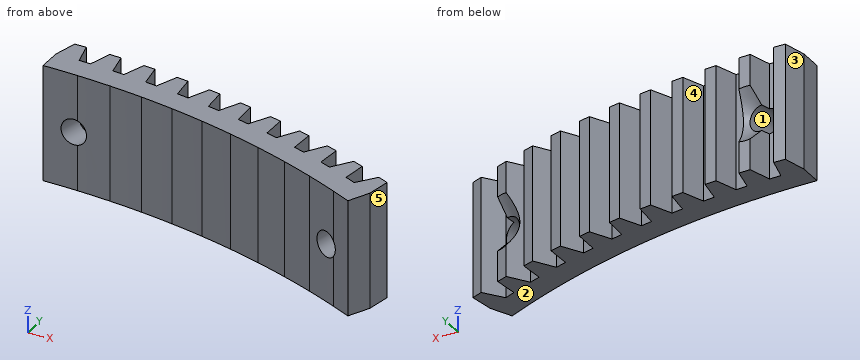
from build123d import *

# Parameters (mm, degrees)
BOSS_EXTRUDE1_DEPTH                                = 25.4
CIRPATTERN2_COUNT                                  = 11
CIRPATTERN2_ANGLE                                  = 23.5
CUT_EXTRUDE2_DEPTH                                 = 25.4
CSK_FOR_10_FLAT_HEAD_MACHINE_SCREW_100_D           = 5.6134
CSK_FOR_10_FLAT_HEAD_MACHINE_SCREW_100_CSINK_D     = 12.7
CSK_FOR_10_FLAT_HEAD_MACHINE_SCREW_100_CSINK_ANGLE = 90


with BuildPart() as part:
    # Sketch1 → Boss-Extrude1 (new body)
    with BuildSketch(Plane.XY):
        with BuildLine():
            Line((1.27, 190.5), (0, 185.42))
            Line((0, 185.42), (0, 180.34))
            ThreePointArc((0, 180.34), (3.828563565, 180.299355798), (7.655401402, 180.177441511))
            Line((7.655401402, 180.177441511), (7.874, 185.32237567))
            ThreePointArc((7.874, 185.32237567), (6.477183927, 185.376451817), (5.08, 185.42))
            Line((5.08, 185.42), (3.81, 190.5))
            Line((3.81, 190.5), (1.27, 190.5))
        make_face()
    boss_extrude1 = extrude(amount=BOSS_EXTRUDE1_DEPTH)

    # CirPattern2: Boss-Extrude1 ×11 about axis
    cirpattern2_axis = Axis((0, 0, 0), (0, 0, -1))
    for i in range(1, CIRPATTERN2_COUNT):
        add(boss_extrude1.rotate(cirpattern2_axis, i * CIRPATTERN2_ANGLE / (CIRPATTERN2_COUNT - 1)))

    # Sketch4 → Cut-Extrude2 (cut)
    with BuildSketch(Plane.XY.offset(25.4)):
        with BuildLine():
            Line((78.866050023, 162.180953733), (81.118055775, 166.812001449))
            ThreePointArc((81.118055775, 166.812001449), (79.858654337, 167.418571633), (78.594717538, 168.015633722))
            Line((78.594717538, 168.015633722), (76.34244866, 163.384044914))
            ThreePointArc((76.34244866, 163.384044914), (77.606580732, 162.787389644), (78.866050023, 162.180953733))
        make_face()
    extrude(amount=-CUT_EXTRUDE2_DEPTH, mode=Mode.SUBTRACT)

    # CSK for _10 Flat Head Machine Screw _100 (through all)
    with Locations(Plane(origin=(40.80368391, 183.714401712, 0), x_dir=(-0.976211516, 0.216820379, 0), z_dir=(0.216820379, 0.976211516, 0))):
        with Locations((-32.344274852, 12.7), (32.394112766, 12.7)):
            CounterSinkHole(CSK_FOR_10_FLAT_HEAD_MACHINE_SCREW_100_D / 2, CSK_FOR_10_FLAT_HEAD_MACHINE_SCREW_100_CSINK_D / 2, counter_sink_angle=CSK_FOR_10_FLAT_HEAD_MACHINE_SCREW_100_CSINK_ANGLE)


solid = part.part
Input: part model. Units: mm. Frame: model coordinates. Face numbers are marked on the shaded views. A direction names the side the tool comes from. Coordinates: 2 decimals unless noted, no trailing zeros. Order: outer loops, then holes, each group sorted by start corner. A loop starts at its lowest first (then second) coordinate and runs counter-clockwise, first axis right, second up.
1. Access query for the marked faces 4 and 5. Directions: +Z, -Z, +X, -X, +Y, -Y. A direction counts if a zero-diameter tool reaches every point of the face in a straight line with its end or side. Return the directions, or none.
Checked values:
face 4: +Z, -Z, +Y
face 5: +Z, -Z, +X, -Y
2. Cut plane B-B, the plane x = 34. Return loops of the section in (y, z), plus the area to 3 significant figures.
Checked values:
outline: (177.11, 0) - (187.46, 0) - (187.46, 25.4) - (177.11, 25.4) - close
area: 263 mm2
3. Contact query for flat-ended pins moving along their axis: P1, Ø4, axis at x = 54, y = 184.5, coming from the +Z side (1 decimal); P2, Ø3, axis at y = 167, z = 7.5, coming from the +X side; P3, Ø8, axis at x = 47.5, z = 5.5, coming from the +Y side; P4, Ø3, axis at y = 180.5, z = 9.5, coming from the -X side. Output: stop coordinate, or through.
Checked values:
P1: passes through
P2: stops at x = 78.68
P3: stops at y = 184.45
P4: stops at x = 0
4. Draft query along Z for the marked faces 1, 2 and 3. Return one class per face: +Z half, -Z half, draft (parallel to the pull), parting line (faces both ways), or undercut.
Checked values:
face 1: undercut
face 2: -Z half
face 3: draft
5. Cut plane A-A, the plane z = 13.5. Count the separate pieces of the cut face and the enclosed holes in it, plus the area to 3 significant figures.
Checked values:
separate pieces: 3
enclosed holes: 0
area: 534 mm2
6. Ray query, line 1 along X through (y, z) = (184.75, 20); line 2 along X through (y, z) = (188, 21.25) (3 decimals); line 3 along Y through (x, z) = (65.5, 9). Return the intervals inside material, ascending.
Checked values:
line 1: x = 0 to 20.2, 23.04 to 27.63, 31.07 to 35.08, 39.31 to 42.56
line 2: x = 0.645 to 4.435, 8.407 to 12.07, 16.28 to 19.661, 24.293 to 27.235
line 3: y = 168.02 to 173.54
